Here's how the part is built. I have some questions about the finished solid (model axes, mm). A direction names the side the tool comes from. Coordinates: 2 decimals unless noted, no trailing zeros. Write each loop counter-clockwise with the first axis right and the second up, starting at its lowest first coordinate (ties: lowest second). Pieces come first, ordered by that corner, then holes. Notation, with made-up numbers: (42.25, -24.5) -> (56.25, -24.5) arc R11 ccw to (56.25, -4.5) -> close; hole circle Ø6 at (29, 28.25). An arc over 180 degrees is marked (long way). Answer in a Markdown table with one row per item. Add a question column.
from build123d import *

# Parameters (mm, degrees)
BOSS_EXTRUDE1_DEPTH = 6.35
SKETCH2_W           = 3.429
SKETCH2_H           = 25.654
CUT_EXTRUDE1_DEPTH  = 7.35
SKETCH3_R           = 3.175
CUT_EXTRUDE2_DEPTH  = 7.35


with BuildPart() as part:
    # Sketch1 → Boss-Extrude1 (new body)
    with BuildSketch(Plane(origin=(0, 0, 0), x_dir=(1, 0, 0), z_dir=(0, 1, 0))):
        Polygon((-31.75, 0), (31.75, 0), (31.75, 203.2), (82.55, 298.45), (-82.55, 298.45), (-31.75, 203.2), align=None)
    extrude(amount=BOSS_EXTRUDE1_DEPTH)

    # Sketch2 → Cut-Extrude1 (cut, through all)
    with BuildSketch(Plane(origin=(0, 6.35, 0), x_dir=(1, 0, 0), z_dir=(0, 1, 0))):
        with Locations((-17.7165, 44.45)):
            Rectangle(SKETCH2_W, SKETCH2_H)
        with Locations((-17.7165, 118.11)):
            Rectangle(SKETCH2_W, SKETCH2_H)
        with Locations((-17.7165, 191.77)):
            Rectangle(SKETCH2_W, SKETCH2_H)
        with Locations((17.7165, 191.77)):
            Rectangle(SKETCH2_W, SKETCH2_H)
        with Locations((17.7165, 118.11)):
            Rectangle(SKETCH2_W, SKETCH2_H)
        with Locations((17.7165, 44.45)):
            Rectangle(SKETCH2_W, SKETCH2_H)
    extrude(amount=-CUT_EXTRUDE1_DEPTH, mode=Mode.SUBTRACT)

    # Sketch3 → Cut-Extrude2 (cut, through all)
    with BuildSketch(Plane(origin=(0, 6.35, 0), x_dir=(1, 0, 0), z_dir=(0, 1, 0))):
        with Locations((-22.606, 163.83)):
            Circle(SKETCH3_R)
        with Locations((-22.606, 151.13)):
            Circle(SKETCH3_R)
        with Locations((22.606, 151.13)):
            Circle(SKETCH3_R)
        with Locations((22.606, 163.83)):
            Circle(SKETCH3_R)
        with Locations((22.606, 85.09)):
            Circle(SKETCH3_R)
        with Locations((22.606, 72.39)):
            Circle(SKETCH3_R)
        with Locations((-22.606, 72.39)):
            Circle(SKETCH3_R)
        with Locations((-22.606, 85.09)):
            Circle(SKETCH3_R)
    extrude(amount=-CUT_EXTRUDE2_DEPTH, mode=Mode.SUBTRACT)


solid = part.part
Q1. If we mould it in two halves opening along X, with no side actions, what happens to faces 1 (the flat face through (-31.75, 3, -103)), 2 (the flat face through (-16.002, 3, -192)), 3 (the flat face through (0, 3, 0))? For each: pulls with the +X half, pulls with the -X half, needs draft (parallel to the pull), parting line crosses it, or undercut.
Q2. Imagine slicing it at B-B on z = -151.13. Please give me the cut outline in (x, y), plus the area to 3 significant figures.
Q3. I'm going to push flat-ended pins straight in: P1, Ø10, axis at x = 22.606, z = -151.13, coming from the -Y side; P2, Ø1.9, axis at y = 2, z = -116.5, coming from the -X side; P3, Ø2, axis at y = 2.5, z = -43, coming from the +X side; P4, Ø4, axis at x = -22.606, z = -163.83, coming from the +Y side. Where does each tip first touch, or does it pass through?
Q4. Imagine slicing it at D-D on x = -47. Please give me the cut outline in (y, z).
Q5. For faces 4 (the flat face through (19.431, 3, -192)), 5 (the flat face through (31.75, 3, -100)), 6 (the flat face through (1, 3, -298.45)), which set-ups out of +Z, -Z, +X, -X, +Y, -Y let a thin tool reach every point of the face, with its end or its side?
Q6. I need wall thicknesses on line 1 (X direction, y = 4.5, z = -72.39); line 2 (X direction, y = 1, z = -184.5); line 3 (Z direction, x = 22.5, y = 5.5). Which ranges of each line are inside material? Lowest first, please. Write a range as [from, to].
Q7. Imagine slicing it at C-C on y = 3. State how many separate pieces and enclosed holes the cut face has, plus the area to 3 significant figures.
Q8. Imagine slicing it at A-A on z = -43. Please give me the cut outline in (x, y).
Result sheet:
| question | item | result |
|---|---|---|
| 1 | face 1 | pulls with the -X half |
| 1 | face 2 | undercut |
| 1 | face 3 | needs draft |
| 2 | outline | (-31.75, 0) -> (-25.78, 0) -> (-25.78, 6.35) -> (-31.75, 6.35) -> close; (-19.43, 0) -> (19.43, 0) -> (19.43, 6.35) -> (-19.43, 6.35) -> close; (25.78, 0) -> (31.75, 0) -> (31.75, 6.35) -> (25.78, 6.35) -> close |
| 2 | area | 323 mm^2 |
| 3 | P1 | stops at y = 0 |
| 3 | P2 | stops at x = -31.75 |
| 3 | P3 | stops at x = 31.75 |
| 3 | P4 | passes through |
| 4 | outline | (0, -298.45) -> (6.35, -298.45) -> (6.35, -231.79) -> (0, -231.79) -> close |
| 5 | face 4 | +Y, -Y |
| 5 | face 5 | +Z, +X, +Y, -Y |
| 5 | face 6 | -Z, +X, -X, +Y, -Y |
| 6 | line 1 | x = [-31.75, -25.78], [-19.43, 19.43], [25.78, 31.75] |
| 6 | line 2 | x = [-31.75, -19.43], [-16, 16], [19.43, 31.75] |
| 6 | line 3 | z = [-298.45, -167], [-160.66, -154.3], [-147.96, -88.26], [-81.92, -75.56], [-69.22, 0] |
| 7 | separate pieces | 1 |
| 7 | enclosed holes | 14 |
| 7 | area | 23,000 mm^2 |
| 8 | outline | (-31.75, 0) -> (-19.43, 0) -> (-19.43, 6.35) -> (-31.75, 6.35) -> close; (-16, 0) -> (16, 0) -> (16, 6.35) -> (-16, 6.35) -> close; (19.43, 0) -> (31.75, 0) -> (31.75, 6.35) -> (19.43, 6.35) -> close |
